Part model, mm, in its own coordinate system. A direction names the side the tool comes from. Round coordinates to 2 decimals unless told otherwise and drop trailing zeros. Write each loop counter-clockwise with the first axis right and the second up, starting at its lowest first coordinate (ties: lowest second). Pieces come first, ordered by that corner, then holes. Notation, with made-up numbers: M -17,-11 L 20,-11 A3 cw 20,-7 Z; hole C 14,-12 d6. An arc over 180 degrees is marked long. Use a Markdown table: item, result. Add a question column.
1) Slice it at B-B on z = 1.2. Give the number of separate pieces and of enclosed holes in the cut face, plus the area to 3 significant figures.
2) Drop flat-ended pins along their axis: P1, Ø1, axis at x = -66.5, z = 2.5, coming from the +Y side; P2, Ø1, axis at y = -21.5, z = 2, coming from the +X side; P3, Ø1, axis at x = 1.5, z = 1.5, coming from the -Y side. Give the stop position or say it passes through.
3) Two-plate mould, pull along Y, no slides. Class faces 1 (the face through (2, -30, 2)), 2 (the face through (-61, 3.175, 2)), 3 (the face through (-101.6, -13, 2)): released by +Y, released by -Y, zero draft, split by the parting line, or undercut.
4) Wall check: probe 1 along Y at (x, z) = (-25.4, 1.3); probe 2 along Y at (x, z) = (-88.5, 2.05); probe 3 along X at (y, z) = (-31.5, 0.8). Give the ranges that are in metal, low to high.
5) Slice it at C-C on y = -14. Write the cut outline in (x, z) (3 decimals).
6) Which spindle directions (+Z, -Z, +X, -X, +Y, -Y) get a long thin tool onto all of the face, cutting with end or side? Do faces 4 (the face through (2, -15, 2)), 5 (the face through (-101.6, -23, 2)), 6 (the face through (-56, 0, 2)). Say none if no direction does.
7) Slice it at A-A on x = -25.4. Write the cut outline in (y, z) (3 decimals).
```python
from build123d import *

# Parameters (mm, degrees)
SKETCH1_R           = 2.5
BOSS_EXTRUDE1_DEPTH = 3.175


with BuildPart() as part:
    # Sketch1 → Boss-Extrude1 (new body)
    with BuildSketch(Plane.XY):
        Polygon((-101.6, 0), (-83.3, 0), (-83.3, 3.175), (-78.3, 3.175), (-78.3, 0), (-73.3, 0), (-73.3, 3.175), (-68.3, 3.175), (-68.3, 0), (-63.3, 0), (-63.3, 3.175), (-58.3, 3.175), (-58.3, 0), (-53.3, 0), (-53.3, 3.175), (-48.3, 3.175), (-48.3, 0), (-43.3, 0), (-43.3, 3.175), (-38.3, 3.175), (-38.3, 0), (-33.3, 0), (-33.3, 3.175), (-28.3, 3.175), (-28.3, 0), (-23.3, 0), (-23.3, 3.175), (-18.3, 3.175), (-18.3, 0), (0, 0), (0, -5), (3.175, -5), (3.175, -10), (0, -10), (0, -15), (3.175, -15), (3.175, -20), (0, -20), (0, -25), (3.175, -25), (3.175, -30), (0, -30), (0, -38.1), (-101.6, -38.1), (-101.6, -30), (-104.775, -30), (-104.775, -25), (-101.6, -25), (-101.6, -20), (-104.775, -20), (-104.775, -15), (-101.6, -15), (-101.6, -10), (-104.775, -10), (-104.775, -5), (-101.6, -5), align=None)
        with Locations((-76.2, -25.4)):
            Circle(SKETCH1_R, mode=Mode.SUBTRACT)
        with Locations((-25.4, -25.4)):
            Circle(SKETCH1_R, mode=Mode.SUBTRACT)
    extrude(amount=BOSS_EXTRUDE1_DEPTH)


solid = part.part
```
Entries:
| question | item | result |
|---|---|---|
| 1 | separate pieces | 1 |
| 1 | enclosed holes | 2 |
| 1 | area | 4,040 mm^2 |
| 2 | P1 | stops at y = 0 |
| 2 | P2 | stops at x = 0 |
| 2 | P3 | stops at y = -30 |
| 3 | face 1 | released by -Y |
| 3 | face 2 | released by +Y |
| 3 | face 3 | undercut |
| 4 | probe 1 | y = -38.1 to -27.9, -22.9 to 0 |
| 4 | probe 2 | y = -38.1 to 0 |
| 4 | probe 3 | x = -101.6 to 0 |
| 5 | outline | M -101.6,0 L 0,0 L 0,3.175 L -101.6,3.175 Z |
| 6 | face 4 | +Z, -Z, +X |
| 6 | face 5 | +Z, -Z, -X |
| 6 | face 6 | +Z, -Z, +Y |
| 7 | outline | M -38.1,0 L -27.9,0 L -27.9,3.175 L -38.1,3.175 Z; M -22.9,0 L 0,0 L 0,3.175 L -22.9,3.175 Z |
